Geometry: see drawing. Coordinates: mm, zero at the bounding-box minimum. Give positions to 0.01 mm unless a question says otherwise; leave off trailing zeros. Write each loop counter-clockwise with the first axis right and the second up, starting at its lowest first coordinate (ties: lowest second). Pieces come first, ordered by that corner, then holes.
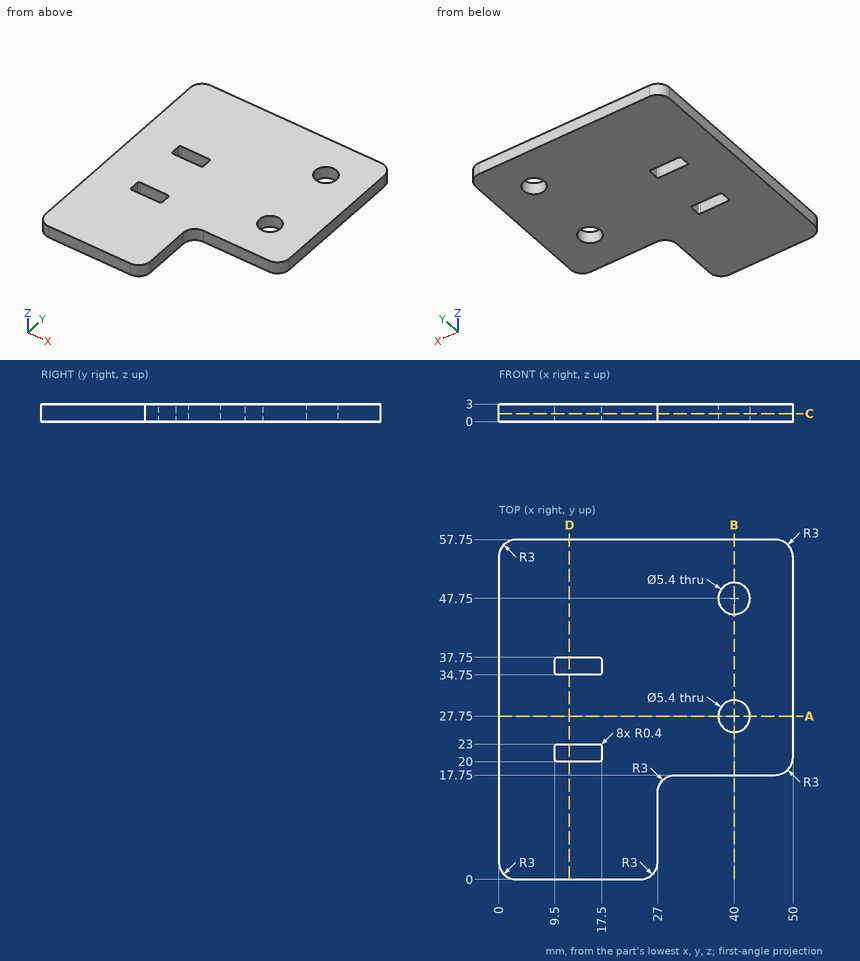
Q1. Pin query (flat end, axial travel): pin 1 (1.5 mm diameter, centred on y = 11.5, z = 1, fed in from +X). Return the tip coordinate at first contact, or that it passes through.
Q2. Material intervals for line 1 along Y through (x, z) = (14, 0.4); line 2 along Y through (x, z) = (40, 1.7); line 3 along X through (y, z) = (21, 1.45), sorted ascending.
Q3. Section B-B, the plane x = 40. Return the cut outline in (y, z), then the cut area to 3 significant figures.
Q4. Section C-C, the plane z = 1.35. Give the number of separate pieces and of enclosed holes in the cut face, then the cut area to 3 significant figures.
Q5. Section D-D, the plane x = 12. Return the cut outline in (y, z).
Q6. Section A-A, the plane y = 27.75. Return the cut outline in (x, z).
Solutions:
1. pin 1: stops at x = 27
2. line 1: y = 0 to 20, 23 to 34.75, 37.75 to 57.75
2. line 2: y = 17.75 to 25.05, 30.45 to 45.05, 50.45 to 57.75
2. line 3: x = 0 to 9.5, 17.5 to 50
3. outline: (17.75, 0) - (25.05, 0) - (25.05, 3) - (17.75, 3) - close; (30.45, 0) - (45.05, 0) - (45.05, 3) - (30.45, 3) - close; (50.45, 0) - (57.75, 0) - (57.75, 3) - (50.45, 3) - close
3. area: 87.6 mm2
4. separate pieces: 1
4. enclosed holes: 4
4. area: 2,380 mm2
5. outline: (0, 0) - (20, 0) - (20, 3) - (0, 3) - close; (23, 0) - (34.75, 0) - (34.75, 3) - (23, 3) - close; (37.75, 0) - (57.75, 0) - (57.75, 3) - (37.75, 3) - close
6. outline: (0, 0) - (37.3, 0) - (37.3, 3) - (0, 3) - close; (42.7, 0) - (50, 0) - (50, 3) - (42.7, 3) - close
